from build123d import *

# Parameters (mm, degrees)
SKETCH1_R           = 4
SKETCH1_R_2         = 3
BOSS_EXTRUDE1_DEPTH = 35
SKETCH1_3_R         = 3
BOSS_EXTRUDE2_DEPTH = 25
FILLET1_R           = 4


with BuildPart() as part:
    # Sketch1 → Boss-Extrude1 (new body)
    # profile 1 of 2: a face of its own
    with BuildSketch(Plane(origin=(0, 0, 0), x_dir=(1, 0, 0), z_dir=(0, 1, 0))):
        with Locations(Location((0, 0, 0), (0, 0, 270))):
            Circle(SKETCH1_R)
    # profile 2 of 2: a face of its own
    with BuildSketch(Plane(origin=(0, 0, 0), x_dir=(1, 0, 0), z_dir=(0, 1, 0))):
        with Locations(Location((0, 0, 0), (0, 0, 270))):
            Circle(SKETCH1_R)
        Circle(SKETCH1_R_2, mode=Mode.SUBTRACT)
    extrude(amount=BOSS_EXTRUDE1_DEPTH)

    # Sketch1_3 → Boss-Extrude2 (add)
    with BuildSketch(Plane(origin=(0, 0, 0), x_dir=(1, 0, 0), z_dir=(0, 1, 0))):
        with Locations(Location((0, 0, 0), (0, 0, 270))):
            Circle(SKETCH1_3_R)
    extrude(amount=-BOSS_EXTRUDE2_DEPTH)

    # Fillet1
    fillet1_edges = [part.edges().sort_by_distance(p)[0] for p in [
        (0, 35, -4),
    ]]
    fillet(fillet1_edges, radius=FILLET1_R)


solid = part.part
Work out the finished part from the listing and answer in its coordinate system (mm). A direction names the side the tool comes from. Round coordinates to 2 decimals unless told otherwise and drop trailing zeros. Loops run counter-clockwise (first coordinate to the right, second up) from the corner with the lowest first, then second, coordinate; pieces in that order, holes last. Notation, with made-up numbers: (-4, 3) - (19, 3) arc R25 ccw to (19, 27) - close; hole circle Ø4 at (81, 39). An arc over 180 degrees is marked (long way). Use one line per item in the form item = value. Start each with the question number.
(1) Find section C-C on y = -21. Determine the outline of the cut face in (x, z), and give its area (3 significant figures).
(2) Which of the six approach directions +Z, -Z, +X, -X, +Y, -Y give full straight-line access (tool end or side, diameter ignored) to faces 1 (the face through (0.9, -12.32, 2.86)), 2 (the face through (0, -25, 0))?
(3) Find section D-D on y = 1. Determine the outline of the cut face in (x, z), and give its area (3 significant figures).
(4) Find section B-B on z = 0. Determine the outline of the cut face in (x, y), and give its area (3 significant figures).
(5) Consider line 1 (Z direction, x = -0.25, y = -6.5); line 2 (X direction, y = 9.5, z = 0.25). Determine where each line is inside the solid, lowest interval first.
(6) Find section A-A on x = 0. Determine the outline of the cut face in (y, z).
(7) Flat-ended cylindrical pins translate along their axes: P1, Ø4, axis at x = 2, z = -1.5, coming from the +Y side; P2, Ø4, axis at x = 1, y = 22.5, coming from the +Z side; P3, Ø4, axis at x = -3, y = -5.5, coming from the +Z side; P4, Ø3, axis at y = 15.5, z = 3, coming from the -X side. Find the tip coordinate at first contact, or state that the pin passes through.
Answer list:
q1.outline = circle Ø6 at (0, 0)
q1.area = 28.3 mm^2
q2.face_1 = -Y
q2.face_2 = +Z, -Z, +X, -X, -Y
q3.outline = circle Ø8 at (0, 0)
q3.area = 50.3 mm^2
q4.outline = (-4, 0) - (-3, 0) - (-3, -25) - (3, -25) - (3, 0) - (4, 0) - (4, 31) arc R4 ccw to (-4, 31) - close
q4.area = 423 mm^2
q5.line_1 = -2.99 to 2.99
q5.line_2 = -3.99 to 3.99
q6.outline = (-25, -3) - (0, -3) - (0, -4) - (31, -4) arc R4 ccw to (31, 4) - (0, 4) - (0, 3) - (-25, 3) - close
q7.P1 = 34.97
q7.P2 = 4
q7.P3 = 2.83
q7.P4 = -3.71
